Part model, mm, in its own coordinate system. A direction names the side the tool comes from. Give positions to 0.01 mm unless a question says otherwise; leave off trailing zeros. Loops run counter-clockwise (first coordinate to the right, second up) from the corner with the lowest first, then second, coordinate; pieces in that order, holes last. Notation, with made-up numbers: (39.25, 53.5) -> (80.25, 53.5) arc R33 cw to (80.25, 86.5) -> close; hole circle Ø1 at (6, -14.5). An arc over 180 degrees is marked (long way). One line per question, with ' | ' between items.
```python
from build123d import *

# Parameters (mm, degrees)
F0_R     = 13.155886
F0_R_2   = 7.519741
F0_R_3   = 21.320013
F1_DEPTH = 25.4
F2_R     = 32.685554
F2_R_2   = 21.320013
F3_DEPTH = 50.8


with BuildPart() as f1:
    # F0 (on Top) → F1 (new body)
    with BuildSketch(Plane.XY):
        with BuildLine():
            ThreePointArc((-156.815305, 20.465674), (-141.271435, 15.07379), (-134.678623, 0))
            ThreePointArc((-134.678623, 0), (-141.271435, -15.07379), (-156.815305, -20.465674))
            Line((-156.815305, -20.465674), (-43.91796, -29.33575))
            ThreePointArc((-43.91796, -29.33575), (-12.40194, -35.904827), (16.449735, -50.187445))
            Line((16.449735, -50.187445), (43.889078, -68.430968))
            ThreePointArc((43.889078, -68.430968), (39.777248, -35.824191), (72.635041, -36.513003))
            Line((72.635041, -36.513003), (25.182848, 20.836736))
            ThreePointArc((25.182848, 20.836736), (30.752729, 11.073168), (32.685554, 0))
            ThreePointArc((32.685554, 0), (-22.188577, -24.000259), (-2.560137, 32.585136))
            Line((-2.560137, 32.585136), (-156.815305, 20.465674))
        make_face()
        with BuildLine():
            ThreePointArc((-156.815305, -20.465674), (-141.271435, -15.07379), (-134.678623, 0))
            ThreePointArc((-134.678623, 0), (-141.271435, 15.07379), (-156.815305, 20.465674))
            ThreePointArc((-156.815305, 20.465674), (-175.736109, 0), (-156.815305, -20.465674))
        make_face()
        with Locations((-155.207366, 0)):
            Circle(F0_R, mode=Mode.SUBTRACT)
        with BuildLine():
            ThreePointArc((77.618277, -50.352592), (76.334511, -42.997885), (72.635041, -36.513003))
            ThreePointArc((72.635041, -36.513003), (39.777248, -35.824191), (43.889078, -68.430968))
            ThreePointArc((43.889078, -68.430968), (66.164518, -69.486897), (77.618277, -50.352592))
        make_face()
        with Locations((55.9088, -50.352592)):
            Circle(F0_R_2, mode=Mode.SUBTRACT)
        with BuildLine():
            ThreePointArc((25.182848, 20.836736), (12.745705, 30.098047), (-2.560137, 32.585136))
            ThreePointArc((-2.560137, 32.585136), (-22.188577, -24.000259), (32.685554, 0))
            ThreePointArc((32.685554, 0), (30.752729, 11.073168), (25.182848, 20.836736))
        make_face()
        Circle(F0_R_3, mode=Mode.SUBTRACT)
    extrude(amount=F1_DEPTH)

    # F2 (on face) → F3 (join)
    with BuildSketch(Plane.XY.offset(25.4)):
        Circle(F2_R)
        Circle(F2_R_2, mode=Mode.SUBTRACT)
    extrude(amount=F3_DEPTH)


solid = f1.part
```
1) Drill centre lines: line 1 (X direction, y = 6, z = 8); line 2 (X direction, y = -7, z = 6.5); line 3 (Y direction, x = 0, z = 48). Where is each one in solid material? Low to high.
Found:
line 1: -174.84 to -166.92, -143.5 to -20.46, 20.46 to 37.46 | line 2: -174.51 to -166.35, -144.07 to -20.14, 20.14 to 48.22 | line 3: -32.69 to -21.32, 21.32 to 32.69
2) Saw through at C-C (x = 0). Give the cut face in (y, z), and give its area (3 significant figures).
Found:
outline: (-40.93, 0) -> (-21.32, 0) -> (-21.32, 76.2) -> (-32.69, 76.2) -> (-32.69, 25.4) -> (-40.93, 25.4) -> close; (21.32, 0) -> (32.69, 0) -> (32.69, 76.2) -> (21.32, 76.2) -> close | area: 1,940 mm2
3) Saw through at B-B (y = 0). Give the cut face in (x, z), and give its area (3 significant figures).
Found:
outline: (-175.74, 0) -> (-168.36, 0) -> (-168.36, 25.4) -> (-175.74, 25.4) -> close; (-142.05, 0) -> (-21.32, 0) -> (-21.32, 76.2) -> (-32.69, 76.2) -> (-32.69, 25.4) -> (-142.05, 25.4) -> close; (21.32, 0) -> (42.42, 0) -> (42.42, 25.4) -> (32.69, 25.4) -> (32.69, 76.2) -> (21.32, 76.2) -> close | area: 4,940 mm2
4) Saw through at A-A (z = 5.5). Give the cut face in (x, y).
Found:
outline: (-156.82, -20.47) -> (-43.92, -29.34) arc R127 cw to (16.45, -50.19) -> (43.89, -68.43) arc R21.71 ccw to (77.62, -50.35) arc R21.71 ccw to (72.64, -36.51) -> (25.18, 20.84) arc R32.69 ccw to (-2.56, 32.59) -> (-156.82, 20.47) arc R20.53 ccw to start; hole circle Ø26.31 at (-155.21, 0); hole circle Ø42.64 at (0, 0); hole circle Ø15.04 at (55.91, -50.35)
5) Saw through at D-D (z = 71). Give the cut face in (x, y), and give its area (3 significant figures).
Found:
outline: circle Ø65.37 at (0, 0); hole circle Ø42.64 at (0, 0) | area: 1,930 mm2
6) Tool access for faces 1 (the cylindrical face through (54.3, -57.7, 12.5)), 2 (the cylindrical face through (-32.654, 1.437, 50.444)): list every direction of +Z, -Z, +X, -X, +Y, -Y with a clear straight run to the whole face (end or side of a thin tool).
Found:
face 1: +Z, -Z | face 2: +Z
7) Pin check, flat tips, straight feed: P1, Ø2.5, axis at x = 9, y = 31.5, coming from the -Z side; P2, Ø8, axis at y = -33.5, z = 62.5, coming from the +X side; P3, Ø10, axis at y = 10, z = 16, coming from the -X side; P4, Ø3, axis at y = -29, z = 30.5, coming from the -X side. Stop position of each tip, or through.
Found:
P1: z = 0 | P2: x = 14.07 | P3: x = -175.12 | P4: x = -17.67
